Here's how the part is built. I have some questions about the finished solid (model axes, mm). Face numbers are marked on the shaded views. Give positions to 0.01 mm unless a question says otherwise; leave off trailing zeros. Loops run counter-clockwise (first coordinate to the right, second up) from the corner with the lowest first, then second, coordinate; pieces in that order, holes last. Notation, with made-up numbers: (-25, 88) - (19, 88) arc R18 ccw to (19, 106) - close; hole circle Ø3 at (87, 18.25). An arc over 180 degrees is marked (long way). Return JSON: item names as keys, results as strings. Group by question number.
(1) If we section it at D-D (x = 13): Please give me the cut outline in (y, z).
(2) I need wall thicknesses on probe 1 along Y at (x, z) = (0, 4.2); probe 2 along Z at (x, y) = (7.5, 12); probe 3 along Y at (x, z) = (-10, 2.8). Which ranges of each line are inside material? Lowest first, please. Write a range as [from, to].
(3) If we section it at A-A (y = 0): Please give me the cut outline in (x, z).
(4) If we section it at B-B (z = 5.6): Please give me the cut outline in (x, y), then the cut area to 3 significant figures.
(5) If we mould it in two halves opening along X, with no side actions, what happens to the marked faces 1, 2, 3 and 4? For each: released by +X, released by -X, zero draft, split by the parting line, or undercut.
(6) For P1, Ø8, axis at x = 0.5, y = 8.5, coming from the +Z side; P2, Ø1, axis at x = 6, z = 2.5, coming from the -Y side (3 decimals); P3, Ø1, axis at y = 7, z = 5, coming from the +X side, each with a flat end and sliding along its axis, tell me the tip position at first contact or that it passes through.
(7) If we section it at C-C (x = -1): Please give me the cut outline in (y, z).
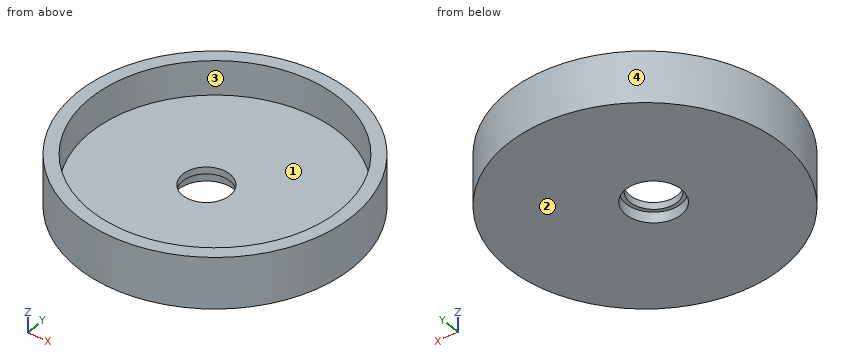
```python
from build123d import *

# Parameters (mm, degrees)
SKETCH1_R           = 16
BOSS_EXTRUDE1_DEPTH = 6
SKETCH3_R           = 14.5
CUT_EXTRUDE1_DEPTH  = 4
SKETCH4_R           = 2.75
CUT_EXTRUDE2_DEPTH  = 2
SKETCH6_R           = 3.25
CUT_EXTRUDE3_DEPTH  = 1.2
DRAFT4_ANGLE        = 3


with BuildPart() as part:
    # Sketch1 → Boss-Extrude1 (new body)
    with BuildSketch(Plane.XY):
        Circle(SKETCH1_R)
    extrude(amount=BOSS_EXTRUDE1_DEPTH)

    # Sketch3 → Cut-Extrude1 (cut)
    with BuildSketch(Plane.XY.offset(6)):
        Circle(SKETCH3_R)
    extrude(amount=-CUT_EXTRUDE1_DEPTH, mode=Mode.SUBTRACT)

    # Sketch4 → Cut-Extrude2 (cut)
    with BuildSketch(Plane(origin=(0, 0, 0), x_dir=(-1, 0, 0), z_dir=(0, 0, -1))):
        with Locations((1, 0)):
            Circle(SKETCH4_R)
    extrude(amount=-CUT_EXTRUDE2_DEPTH, mode=Mode.SUBTRACT)

    # Sketch6 → Cut-Extrude3 (cut)
    with BuildSketch(Plane(origin=(0, 0, 0), x_dir=(-1, 0, 0), z_dir=(0, 0, -1))):
        with Locations((1, 0)):
            Circle(SKETCH6_R)
    extrude(amount=-CUT_EXTRUDE3_DEPTH, mode=Mode.SUBTRACT)

    # Draft4
    draft4_faces = [part.faces().sort_by_distance(p)[0] for p in [
        (2.25, 0, 0.6),
    ]]
    draft(draft4_faces, Plane(origin=(0, 0, 0), x_dir=(-1, 0, 0), z_dir=(0, 0, -1)), DRAFT4_ANGLE)


solid = part.part
```
Values:
{
 "1": {"outline": "(-9.33, 0) - (9.33, 0) - (9.33, 6) - (6.42, 6) - (6.42, 2) - (-6.42, 2) - (-6.42, 6) - (-9.33, 6) - close"},
 "2": {"probe 1": "[-16, -14.5], [14.5, 16]", "probe 2": "[0, 2]", "probe 3": "[-12.49, -10.5], [10.5, 12.49]"},
 "3": {"outline": "(-16, 0) - (-4.25, 0) - (-4.19, 1.2) - (-3.75, 1.2) - (-3.75, 2) - (-14.5, 2) - (-14.5, 6) - (-16, 6) - close; (1.75, 1.2) - (2.19, 1.2) - (2.25, 0) - (16, 0) - (16, 6) - (14.5, 6) - (14.5, 2) - (1.75, 2) - close"},
 "4": {"outline": "circle Ø32 at (0, 0); hole circle Ø29 at (0, 0)", "area": "144 mm2"},
 "5": {"face 1": "undercut", "face 2": "zero draft", "face 3": "undercut", "face 4": "split by the parting line"},
 "6": {"P1": "z = 2", "P2": "y = -15.025", "P3": "x = 14.62"},
 "7": {"outline": "(-15.97, 0) - (-3.25, 0) - (-3.19, 1.2) - (-2.75, 1.2) - (-2.75, 2) - (-14.47, 2) - (-14.47, 6) - (-15.97, 6) - close; (2.75, 1.2) - (3.19, 1.2) - (3.25, 0) - (15.97, 0) - (15.97, 6) - (14.47, 6) - (14.47, 2) - (2.75, 2) - close"}
}
